from build123d import *

# Parameters (mm, degrees)
F2_R     = 3.75
F3_DEPTH = 1
F4_W     = 5.9792066569
F4_H     = 4.5275918273
F5_DEPTH = 3
F6_DEPTH = 5


# Not quite as in the source:
# - the program builds the solid bodies; features that only make, move or delete a surface that nothing else refers to are left out


with BuildPart() as f3:
    # F2 (on Top) → F3 (new body)
    with BuildSketch(Plane.XY):
        Circle(F2_R)
    extrude(amount=F3_DEPTH)

    # F4 (on face) → F5 (join)
    with BuildSketch(Plane(origin=(0, 0, 0), x_dir=(1, 0, 0), z_dir=(0, 0, -1))):
        Rectangle(F4_W, F4_H)
    extrude(amount=F5_DEPTH)

    # F6 (add): a face of the model
    f6_faces = [f3.faces().sort_by_distance(p)[0] for p in [
        (0, 0, -3),
    ]]
    extrude(f6_faces, amount=F6_DEPTH)


solid = f3.part
The listing builds one solid part. Answer for the finished solid, in the listing's coordinates (mm). A direction names the side the tool comes from. Give positions to 0.01 mm unless a question says otherwise; leave off trailing zeros. Write each loop counter-clockwise with the first axis right and the second up, starting at its lowest first coordinate (ties: lowest second). Pieces come first, ordered by that corner, then holes. Notation, with made-up numbers: (-13, -32.75) - (-3, -32.75) arc R21 cw to (-3, -9.75) - close; hole circle Ø3 at (25.5, 83). An arc over 180 degrees is marked (long way). Use a Markdown table: item, result.
1. Each of these flat-tipped pins is pushed along its axis until it touches: P1, Ø1.4, axis at y = -1, z = -5, coming from the -X side; P2, Ø2.5, axis at y = 0.5, z = -5.5, coming from the +X side; P3, Ø1.5, axis at x = 1.5, z = -0.5, coming from the -Y side. Where does it stop, or does it pass through?
Values follow:
| item | result |
|---|---|
| P1 | stops at x = -2.99 |
| P2 | stops at x = 2.99 |
| P3 | stops at y = -3.63 |
2. Section A-A on x = 0 is taken. Write down the section's boundary in (y, z).
Values follow:
| item | result |
|---|---|
| outline | (-3.75, 0) - (-2.26, 0) - (-2.26, -8) - (2.26, -8) - (2.26, 0) - (3.75, 0) - (3.75, 1) - (-3.75, 1) - close |
3. Section C-C on z = -7 is taken. Write down the section's boundary in (x, y).
Values follow:
| item | result |
|---|---|
| outline | (-2.99, -2.26) - (2.99, -2.26) - (2.99, 2.26) - (-2.99, 2.26) - close |
4. Find the intervals of material crossed by probe 1 along Y at (x, z) = (-2.5, -5.5); probe 2 along Z at (x, y) = (1.25, 2.5); probe 3 along X at (y, z) = (-0.25, -3.25), in increasing order. Write a range as from..to.
Values follow:
| item | result |
|---|---|
| probe 1 | y = -2.26..2.26 |
| probe 2 | z = 0..1 |
| probe 3 | x = -2.99..2.99 |
5. A tool of negligible diameter and unlimited length cuts with its end or side. For faces 1 (the flat face through (0, -2.264, -4)), 2 (the flat face through (2.99, 0, -4)), 3 (the flat face through (-2.99, 0, -4)), 4 (the flat face through (0, 3, 0)), 5 (the flat face through (0, 0, 1)), from which of +Z, -Z, +X, -X, +Y, -Y can it reach the whole face along a straight path? Write none if from no direction.
Values follow:
| item | result |
|---|---|
| face 1 | -Z, +X, -X, -Y |
| face 2 | -Z, +X, +Y, -Y |
| face 3 | -Z, -X, +Y, -Y |
| face 4 | -Z, +X, -X, +Y |
| face 5 | +Z, +X, -X, +Y, -Y |
6. Section B-B on y = 0 is taken. Write down the section's boundary in (x, z), plus the area to 3 significant figures.
Values follow:
| item | result |
|---|---|
| outline | (-3.75, 0) - (-2.99, 0) - (-2.99, -8) - (2.99, -8) - (2.99, 0) - (3.75, 0) - (3.75, 1) - (-3.75, 1) - close |
| area | 55.3 mm² |
7. Section D-D on y = 2.5 is taken. Write down the section's boundary in (x, z).
Values follow:
| item | result |
|---|---|
| outline | (-2.8, 0) - (2.8, 0) - (2.8, 1) - (-2.8, 1) - close |
